Autodesk Inventor part; units mm, degrees
sketch "Sketch1" plane through (0, 0, 0) normal (0, 1, 0) x (-1, 0, 0)
  circle A0 centre (0, 0) radius 37.5
  circle A1 centre (0, 0) radius 25
  dimension "d0" = 75
  dimension "d1" = 50
extrude "Extrusion1" add sketch "Sketch1" along normal blind 540
sketch "Sketch2" plane through (0, 0, 0) normal (0, 1, 0) x (-1, 0, 0)
  line L0 (-37.5, -37.5) -> (37.5, -37.5)
  line L1 (37.5, -37.5) -> (37.5, 37.5)
  line L2 (37.5, 37.5) -> (-37.5, 37.5)
  line L3 (-37.5, 37.5) -> (-37.5, -37.5)
  point P0 (0, 0)
extrude "Extrusion2" add sketch "Sketch2" against normal blind 60
sketch "Sketch3" plane through (0, 0, 0) normal (0, 0, 1) x (1, 0, 0)
  circle A0 centre (0, -30) radius 15
  line L0 (-52.5, 0) -> (52.5, 0)
  line L1 (-37.5, 0) -> (-37.5, -60)
  line L2 (37.5, 0) -> (37.5, -60)
  arc A1 (-37.5, -30) -> (37.5, -30) centre (0, -21.5625) ccw
  line L3 (-37.5, -30) -> (-52.5, -30)
  line L4 (-52.5, -30) -> (-52.5, -80.2965)
  line L5 (-52.5, -80.2965) -> (57.4115, -80.2965)
  line L6 (57.4115, -80.2965) -> (57.4115, -30)
  line L7 (57.4115, -30) -> (37.5, -30)
  point P0 (0, 0)
  dimension "d6" = 30
  dimension "d7" = 30
extrude "Extrusion3" cut sketch "Sketch3" along normal mid plane 150 contours A0 | A1 L7 L6 L5 L4 L3
fillet "Fillet1" radius 37.5 4 edges at (37.5, -15, 37.5) (37.5, -15, -37.5) (-37.5, -15, 37.5) (-37.5, -15, -37.5)
properties part number "Cylinder_Bom"
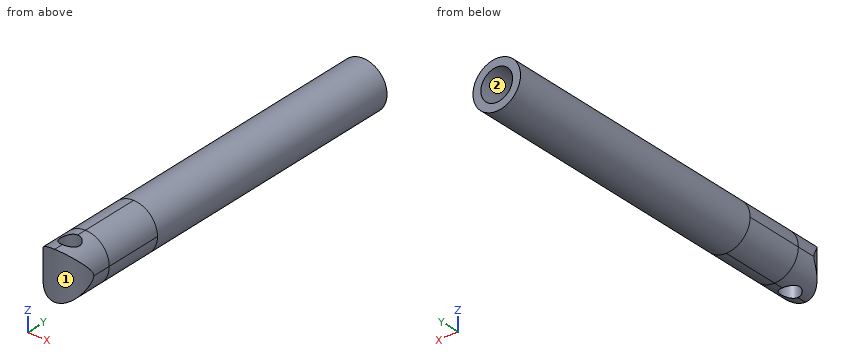
Design review of the part built by this model. Coordinates are the model's own, in mm. Face numbers are marked on the shaded views. Coordinates: 2 decimals unless noted, no trailing zeros. Loops run counter-clockwise (first coordinate to the right, second up) from the corner with the lowest first, then second, coordinate; pieces in that order, holes last. Notation, with made-up numbers: (42.5, 61.25) -> (50.5, 61.25) arc R8 ccw to (50.5, 69.25) -> close; hole circle Ø11 at (27, 84.25). An arc over 180 degrees is marked (long way). Answer as a JSON object with one key per item and string values.
Q1. Take a section at D-D on y = -9. Give the boundary of the cut face in (x, z).
Answer block:
{"outline": "circle Ø75 at (0, 0)"}
Q2. Clearance check with flat-ended pins moving along their axes: pin 1 Ø6 at (y, z) = (258.5, 11.5) entering from -X; pin 2 Ø1.5 at (x, y) = (-17, 72) entering from -Z; pin 3 Ø10 at (x, y) = (25.5, 78) entering from -Z. State where each tip first meets the part, or that it passes through.
Answer block:
{"pin 1": "stops at x = -36.52", "pin 2": "stops at z = -33.8", "pin 3": "stops at z = -31.4"}
Q3. The part is to be moulded in two halves that separate along X. For the marked faces 1 and 2, say which applies: +X half, -X half, draft (parallel to the pull), parting line (faces both ways), or undercut.
Answer block:
{"face 1": "parting line", "face 2": "undercut"}
Q4. Take a section at A-A on x = 9. Give the boundary of the cut face in (y, z).
Answer block:
{"outline": "(-58.93, -36.4) -> (-42, -36.4) -> (-42, 36.4) -> (-58.93, 36.4) -> close; (-18, -36.4) -> (540, -36.4) -> (540, -23.32) -> (0, -23.32) -> (0, 23.32) -> (540, 23.32) -> (540, 36.4) -> (-18, 36.4) -> close"}
Q5. Take a section at B-B on z = 10.5. Give the boundary of the cut face in (x, y) (1 decimal).
Answer block:
{"outline": "(-36, -35) arc R38.4 ccw to (36, -35) -> (36, 540) -> (22.7, 540) -> (22.7, 0) -> (-22.7, 0) -> (-22.7, 540) -> (-36, 540) -> close; hole circle Ø30 at (0, -30)"}
Q6. To check wall thickness, follow L1, parallel to Y at x = 0, z = 28; L2, parallel to Y at x = 0, z = -21.5; L3, parallel to Z at x = 4.5, y = 394.5. State the ranges of each line that lie inside material, in increasing order.
Answer block:
{"L1": "y = -60 to -45, -15 to 540", "L2": "y = -60 to -45, -15 to 0", "L3": "z = -37.23 to -24.59, 24.59 to 37.23"}
Q7. Take a section at C-C on y = 253. Give the boundary of the cut face in (x, z), plus the area to 3 significant figures.
Answer block:
{"outline": "circle Ø75 at (0, 0); hole circle Ø50 at (0, 0)", "area": "2,450 mm^2"}
